Check sheet for the modelled part. Datum: model origin and axes. Units: mm. A direction names the side the tool comes from. Coordinates: 2 decimals unless noted, no trailing zeros. Write each loop counter-clockwise with the first axis right and the second up, starting at its lowest first coordinate (ties: lowest second). Pieces come first, ordered by that corner, then holes. Notation, with made-up numbers: M 62.5,27 L 69.5,27 A33 cw 69.5,66 Z; hole C 36.25,0.25 d4. An arc over 180 degrees is marked long. Answer as CSV lines item,"result". Start each with the question number.
Q1. Mould release check, pull along X, two halves, no side actions. Record for faces 4 (the cylindrical face through (-14.144, -21.922, -0.322)), 5 (the cylindrical face through (-29.97, 1.32, 0.32)), 6 (the cylindrical face through (-19.39, -9.48, -0.32)), 7 (the flat face through (2, 9, -25)): pulls with the +X half, pulls with the -X half, needs draft (parallel to the pull), parting line crosses it, or undercut.
Q2. Sectioned sample at A-A, the plane y = 6. Record the cut outline in (x, z), then the cut area to 3 significant figures.
Q3. Sectioned sample at B-B, the plane z = 15. Count the separate pieces of the cut face and the enclosed holes in it, then the cut area to 3 significant figures.
Q4. Sectioned sample at D-D, the plane x = -20. Record the cut outline in (y, z), then the cut area to 3 significant figures.
Q5. Sectioned sample at C-C, the plane x = 0. Record the cut outline in (y, z).
Q6. Depth check by flat-ended pin: pin 1 Ø4.5 at (x, y) = (20.4, -12.16) entering from -Z; pin 2 Ø8 at (x, y) = (11.59, -20.73) entering from +Z; pin 3 Ø6 at (x, y) = (20.73, 11.59) entering from -Z; pin 4 Ø3 at (y, z) = (13.5, -13) entering from -X. Enter the tip coordinate at first touch or a pass-through.
Q7. Thickness scan on line 1 along Y through (x, z) = (1, -3); line 2 along Y through (x, z) = (23, -15); line 3 along X through (y, z) = (-1.5, 11). Record the ranges inside material, lowest first. Write a range as from..to.
Q8. Access from +Z, -Z, +X, -X, +Y, -Y to the whole of each face (thin tool, end or side, straight path). Record for faces 1 (the cylindrical face through (13.97, -19.98, -0.32)), 2 (the flat face through (0, -13, -23)), 3 (the flat face through (0, -13, 23)).
from build123d import *

# Parameters (mm, degrees)
SKETCH1_R           = 30
SKETCH1_R_2         = 12
SKETCH1_R_3         = 2.5
BOSS_EXTRUDE1_DEPTH = 23
SKETCH2_R           = 12
SKETCH2_R_2         = 9
BOSS_EXTRUDE2_DEPTH = 25


with BuildPart() as part:
    # Sketch1 → Boss-Extrude1 (new body, symmetric)
    with BuildSketch(Plane.XY):
        Circle(SKETCH1_R)
        Circle(SKETCH1_R_2, mode=Mode.SUBTRACT)
        with Locations((0.330787081, 23.747696307)):
            Circle(SKETCH1_R_3, mode=Mode.SUBTRACT)
        with Locations((12.160318169, 20.400714743)):
            Circle(SKETCH1_R_3, mode=Mode.SUBTRACT)
        with Locations((20.731501824, 11.587378139)):
            Circle(SKETCH1_R_3, mode=Mode.SUBTRACT)
        with Locations((23.747696307, -0.330787081)):
            Circle(SKETCH1_R_3, mode=Mode.SUBTRACT)
        with Locations((20.400714743, -12.160318169)):
            Circle(SKETCH1_R_3, mode=Mode.SUBTRACT)
        with Locations((11.587378139, -20.731501824)):
            Circle(SKETCH1_R_3, mode=Mode.SUBTRACT)
        with Locations((-0.330787081, -23.747696307)):
            Circle(SKETCH1_R_3, mode=Mode.SUBTRACT)
        with Locations((-12.160318169, -20.400714743)):
            Circle(SKETCH1_R_3, mode=Mode.SUBTRACT)
        with Locations((-20.731501824, -11.587378139)):
            Circle(SKETCH1_R_3, mode=Mode.SUBTRACT)
        with Locations((-23.747696307, 0.330787081)):
            Circle(SKETCH1_R_3, mode=Mode.SUBTRACT)
        with Locations((-20.400714743, 12.160318169)):
            Circle(SKETCH1_R_3, mode=Mode.SUBTRACT)
        with Locations((-11.587378139, 20.731501824)):
            Circle(SKETCH1_R_3, mode=Mode.SUBTRACT)
    extrude(amount=BOSS_EXTRUDE1_DEPTH, both=True)

    # Sketch2 → Boss-Extrude2 (add, symmetric)
    with BuildSketch(Plane.XY):
        Circle(SKETCH2_R)
        Circle(SKETCH2_R_2, mode=Mode.SUBTRACT)
    extrude(amount=BOSS_EXTRUDE2_DEPTH, both=True)


solid = part.part
Output:
1,face 4,"undercut"
1,face 5,"parting line crosses it"
1,face 6,"undercut"
1,face 7,"needs draft"
2,outline,"M -29.39,-23 L -10.39,-23 L -10.39,-25 L -6.71,-25 L -6.71,25 L -10.39,25 L -10.39,23 L -29.39,23 Z; M 6.71,-25 L 10.39,-25 L 10.39,-23 L 29.39,-23 L 29.39,23 L 10.39,23 L 10.39,25 L 6.71,25 Z"
2,area,"2,120 mm^2"
3,separate pieces,"1"
3,enclosed holes,"13"
3,area,"2,340 mm^2"
4,outline,"M -22.36,-23 L -13.98,-23 L -13.98,23 L -22.36,23 Z; M -9.2,-23 L 9.69,-23 L 9.69,23 L -9.2,23 Z; M 14.63,-23 L 22.36,-23 L 22.36,23 L 14.63,23 Z"
4,area,"1,610 mm^2"
5,outline,"M -30,-23 L -26.23,-23 L -26.23,23 L -30,23 Z; M -21.27,-23 L -12,-23 L -12,-25 L -9,-25 L -9,25 L -12,25 L -12,23 L -21.27,23 Z; M 9,-25 L 12,-25 L 12,-23 L 21.27,-23 L 21.27,23 L 12,23 L 12,25 L 9,25 Z; M 26.23,-23 L 30,-23 L 30,23 L 26.23,23 Z"
6,pin 1,"passes through"
6,pin 2,"stops at z = 23"
6,pin 3,"stops at z = -23"
6,pin 4,"stops at x = -27.5"
7,line 1,"y = -29.98..-25.86, -21.63..-8.94, 8.94..21.34, 26.16..29.98"
7,line 2,"y = -19.26..-2.72, 2.05..10.54, 12.64..19.26"
7,line 3,"x = -29.96..-25.45, -22.05..-8.87, 8.87..21.54, 25.96..29.96"
8,face 1,"+Z, -Z"
8,face 2,"-Z"
8,face 3,"+Z"
